Autodesk Fusion 360 part; units mm, degrees
sketch "Sketch1" plane through (0, 0, 0) normal (0, 0, 1) x (1, 0, 0)
  line L0 (78.2063, 84.3769) -> (241.4063, 84.3769)
  line L1 (241.4063, 84.3769) -> (241.4063, -13.5431)
  line L2 (241.4063, -13.5431) -> (78.2063, -13.5431)
  line L3 (78.2063, -13.5431) -> (78.2063, 84.3769)
  line L4 (74.7063, 87.8669) -> (244.9063, 87.8669)
  line L5 (244.9063, 87.8669) -> (244.9063, -23.3331)
  line L6 (244.9063, -23.3331) -> (74.7063, -23.3331)
  line L7 (74.7063, -23.3331) -> (74.7063, 87.8669)
  line L8 (74.7063, 87.8669) -> (244.9063, 87.8669)
  line L9 (244.9063, 87.8669) -> (244.9063, -33.3331)
  line L10 (244.9063, -33.3331) -> (74.7063, -33.3331)
  line L11 (74.7063, -33.3331) -> (74.7063, 87.8669)
  line L12 (149.8063, -33.3331) -> (169.8063, -33.3331)
  line L13 (169.8063, -33.3331) -> (169.8063, -23.3331)
  line L14 (169.8063, -23.3331) -> (149.8063, -23.3331)
  line L15 (149.8063, -23.3331) -> (149.8063, -33.3331)
  line L16 (71.3063, 91.2669) -> (248.3063, 91.2669)
  line L17 (248.3063, 91.2669) -> (248.3063, -36.7331)
  line L18 (248.3063, -36.7331) -> (71.3063, -36.7331)
  line L19 (71.3063, -36.7331) -> (71.3063, 91.2669)
  line L20 (74.3063, 88.2669) -> (245.3063, 88.2669)
  line L21 (245.3063, 88.2669) -> (245.3063, -23.7331)
  line L22 (245.3063, -23.7331) -> (74.3063, -23.7331)
  line L23 (74.3063, -23.7331) -> (74.3063, 88.2669)
  dimension "d1" = 97.92
  dimension "d2" = 163.2
  dimension "d3" = 170.2
  dimension "d4" = 3.5
  dimension "d5" = 111.2
  dimension "d6" = 3.49
  dimension "d7" = 10
  dimension "d8" = 20
  dimension "d9" = 75.1
  dimension "d11" = -3.4
  dimension "d34" = -0.4
  dimension "d35" = 75.1
extrude "Extrude1" add sketch "Sketch1" against normal blind 1.5 contours L4 L5 L7 L8 L9 L11 L20 L21 L22 L23 | L4 L5 L6 L7 L8 L9 L11 L14 | L6 L11 L15 L22 | L6 L9 L13 L22 | L6 L13 L14 L15 L22 | L10 L11 L15 L22 | L9 L10 L13 L22 | L10 L12 L13 L15 L22 | L16 L17 L18 L19
extrude "Extrude2" add sketch "Sketch1" along normal blind 1.2 contours L10 L11 L15 L22 | L9 L10 L13 L22 | L16 L17 L18 L19
sketch "Sketch2" plane through (71.3063, 0, 0) normal (-1, 0, 0) x (0, -1, 0)
  line L0 (-91.2669, 1.2) -> (-91.2669, -1.5)
  line L1 (-91.2669, -1.5) -> (36.7331, -1.5)
  line L2 (36.7331, -1.5) -> (36.7331, 1.2)
  line L3 (36.7331, 1.2) -> (-91.2669, 1.2)
  line L4 (36.7331, -1.5) -> (33.0912, -1.5)
  line L5 (33.0912, -1.5) -> (33.0912, 2.7)
  line L6 (33.0912, 2.7) -> (36.7331, 2.7)
  line L7 (36.7331, 2.7) -> (36.7331, -1.5)
  line L8 (36.7331, 2.7) -> (38.5941, -4.2455)
  line L9 (36.7331, 2.7) -> (43.6271, 2.7) construction
  line L10 (36.7331, -1.5) -> (39.5381, -1.5)
  line L11 (35.2766, 1.2) -> (42.4884, 1.2)
  dimension "d16" = 1.5
  dimension "d17" = 75
extrude "Extrude3" add sketch "Sketch2" against normal up to surface (177 mm away) contours L2 L7 L8 L10 L11
fillet "Fillet1" radius 3 2 edges at (71.3063, 91.2669, -0.15) (248.3063, 91.2669, -0.15)
sketch "Sketch3" plane through (0, 0, -1.5) normal (0, 0, -1) x (1, 0, 0)
  arc A0 (245.3063, -91.2669) -> (248.3063, -88.2669) centre (245.3063, -88.2669) ccw
  line L0 (248.3063, -88.2669) -> (248.3063, 37.8584)
  line L1 (248.3063, 37.8584) -> (71.3063, 37.8584)
  line L2 (71.3063, 37.8584) -> (71.3063, -88.2669)
  arc A1 (71.3063, -88.2669) -> (74.3063, -91.2669) centre (74.3063, -88.2669) ccw
  line L3 (74.3063, -91.2669) -> (245.3063, -91.2669)
  line L4 (78.2063, 13.5431) -> (241.4063, 13.5431)
  line L5 (241.4063, 13.5431) -> (241.4063, -84.3769)
  line L6 (241.4063, -84.3769) -> (78.2063, -84.3769)
  line L7 (78.2063, -84.3769) -> (78.2063, 13.5431)
  spline S0 degree 5 poles (168.3063, 26.3081) (168.3195, 26.3986) (168.2582, 26.6166) (167.9024, 27.0513) (166.9216, 27.7962) (164.9941, 28.7753) (162.5706, 29.5411) (159.8951, 29.8719) (157.2258, 29.6505) (154.8107, 28.9513) (152.8718, 27.9853) (151.5916, 27.0179) (151.0968, 26.2949) (151.4435, 25.9718) (152.5955, 26.024) (154.4375, 26.2989) (156.7949, 26.5955) (159.4487, 26.7323) (162.1514, 26.6209) (164.6413, 26.3369) (166.6674, 26.0492) (167.7451, 25.9733) (168.179, 26.0739) (168.2931, 26.2177) (168.3063, 26.3081) knots 0 0 0 0 0 0 0.05 0.1 0.15 0.2 0.25 0.3 0.35 0.4 0.45 0.5 0.55 0.6 0.65 0.7 0.75 0.8 0.85 0.9 0.95 1 1 1 1 1 1
  circle A2 centre (171.9063, 22.9918) radius 1.5
  circle A3 centre (147.9063, 22.9919) radius 1.5
  point P0 (159.4063, 29.7363)
  point P1 (151.3063, 26.3081)
  point P2 (159.4063, 26.6713)
  dimension "d22" = 80
  dimension "d23" = 80
  dimension "d24" = 3
  dimension "d25" = 3
  dimension "d26" = 88.1
  dimension "d27" = 88.9
  dimension "d28" = 88.1
  dimension "d29" = 24
  dimension "d30" = 3.6
  dimension "d31" = 0.0001
  dimension "d36" = 3.4
sketch "Sketch4" plane through (0, 0, -1.5) normal (0, 0, -1) x (1, 0, 0)
extrude "Extrude4" cut sketch "Sketch3" against normal blind 0.5 contours S0 | A2 | A3
CAD build for the part. Positions are in the model's coordinates, mm. A direction names the side the tool comes from. Give positions to 0.01 mm unless a question says otherwise; leave off trailing zeros. Write each loop counter-clockwise with the first axis right and the second up, starting at its lowest first coordinate (ties: lowest second). Pieces come first, ordered by that corner, then holes. Notation, with made-up numbers: M 30.5,30.5 L 45.5,30.5 A14 cw 45.5,53.5 Z; hole C 60.5,78 d3. An arc over 180 degrees is marked long. Return JSON: item names as keys, results as strings. Group by question number.
(1) Band-saw the part on D-D (y = -15.5). Give the cut face in (x, z), and give its area (3 significant figures).
(2) 3-axis set-ups, long thin cutter, end or side, ignore diameter. For faces 3 (the face through (146, -25, 1.2)), 4 (the face through (160, -28, -1)): which of +Z, -Z, +X, -X, +Y, -Y reach the whole face in a straight line?
(3) Band-saw the part on B-B (y = -0.5). Give the cut face in (x, z), and give its area (3 significant figures).
(4) Band-saw the part on A-A (x = 112). Give the cut face in (y, z).
(5) Flat gauge pins, fed straight in: pin 1 Ø1.2 at (x, z) = (159, -0.5) entering from -Y; pin 2 Ø1 at (x, z) = (131.5, 0.5) entering from -Y; pin 3 Ø1.5 at (x, y) = (172, -23) entering from -Z; pin 4 Ø1.8 at (x, y) = (171.91, -22.99) entering from +Z. Where does each tip first touch, or does it go through?
(6) Drill centre lines: L1, parallel to X at y = 3, z = 0.15; L2, parallel to X at y = 22.5, z = -1.3; L3, parallel to Z at x = 85.5, y = -15. Where is each one in solid material? Low to high. Write a range as [from, to].
(7) Mould opens along Y. For faces 1 (the face through (153, -17, 0)), 2 (the face through (159, -16, -1.5)) say: pulls with the +Y half, pulls with the -Y half, needs draft (parallel to the pull), parting line crosses it, or undercut.
(8) Band-saw the part on C-C (z = -0.55). Give the cut face in (x, y), and give its area (3 significant figures).
Entries:
{
 "1": {"outline": "M 71.31,-1.5 L 248.31,-1.5 L 248.31,1.2 L 245.31,1.2 L 245.31,0 L 74.31,0 L 74.31,1.2 L 71.31,1.2 Z", "area": "273 mm^2"},
 "2": {"face 3": "+Z, +X, -X, +Y, -Y", "face 4": "-Z"},
 "3": {"outline": "M 71.31,-1.5 L 78.21,-1.5 L 78.21,0 L 74.31,0 L 74.31,1.2 L 71.31,1.2 Z; M 241.41,-1.5 L 248.31,-1.5 L 248.31,1.2 L 245.31,1.2 L 245.31,0 L 241.41,0 Z", "area": "27.9 mm^2"},
 "4": {"outline": "M -37.86,-1.5 L -13.54,-1.5 L -13.54,0 L -23.73,0 L -23.73,1.2 L -37.14,1.2 Z; M 84.38,-1.5 L 91.27,-1.5 L 91.27,1.2 L 88.27,1.2 L 88.27,0 L 84.38,0 Z"},
 "5": {"pin 1": "stops at y = -37.75", "pin 2": "stops at y = -37.46", "pin 3": "stops at z = -1", "pin 4": "stops at z = 1.2"},
 "6": {"L1": "x = [71.31, 74.31], [245.31, 248.31]", "L2": "x = [71.31, 78.21], [241.41, 248.31]", "L3": "z = [-1.5, 0]"},
 "7": {"face 1": "undercut", "face 2": "needs draft"},
 "8": {"outline": "M 71.31,-37.6 L 248.31,-37.6 L 248.31,88.27 A3 ccw 245.31,91.27 L 74.31,91.27 A3 ccw 71.31,88.27 Z; hole M 78.21,-13.54 L 241.41,-13.54 L 241.41,84.38 L 78.21,84.38 Z", "area": "6,830 mm^2"}
}
